Verification items for the finished model (mm, model axes). A direction names the side the tool comes from. Give positions to 0.01 mm unless a question says otherwise; leave off trailing zeros. Order: outer loops, then holes, each group sorted by start corner. A loop starts at its lowest first (then second) coordinate and runs counter-clockwise, first axis right, second up. Notation, with made-up numbers: (63.25, 50.5) -> (109.25, 50.5) arc R22 ccw to (109.25, 82.5) -> close; hole circle Ø7 at (85.5, 61). An arc over 180 degrees is marked (long way). Return JSON: item names as keys, results as strings. Group by question number.
(1) Release check for a two-part mould opening along X. For faces 1 (the face through (104, -14, 0)), 2 (the face through (73, 92.3, 20)) record: pulls with the +X half, pulls with the -X half, needs draft (parallel to the pull), parting line crosses it, or undercut.
(2) Cross-section at B-B on y = -3. Enter the section's corners in (x, z).
(3) Cross-section at A-A on x = 79. Enter the section's corners in (y, z).
(4) Cross-section at C-C on z = 4.5. State how many separate pieces and enclosed holes the cut face has, then the cut area to 3 significant figures.
(5) Tool access check on faces 3 (the face through (118.4, 46, 22)), 4 (the face through (68, 31, 45)). Record the directions out of +Z, -Z, +X, -X, +Y, -Y that give a thin tool (end or side, any length) a straight path to the whole face; none if there is none.
(6) Depth check by flat-ended pin: pin 1 Ø1 at (x, y) = (108.5, 36) entering from +Z. Enter the tip coordinate at first touch or a pass-through.
(7) Thickness scan on line 1 along Y through (x, z) = (73.5, 38); line 2 along X through (y, z) = (68.5, 21.5); line 3 along Z through (x, y) = (43, -6.5). Record the ranges inside material, lowest first.
from build123d import *

# Parameters (mm, degrees)
F1_W     = 152.5
F1_H     = 122.4
F2_DEPTH = 4
F3_DEPTH = 45
F0_W     = 28.1
F0_H     = 28.1
F4_DEPTH = 45.001


with BuildPart() as f2:
    # F1 (on Top) → F2 (new body)
    with BuildSketch(Plane.XY):
        with Locations((74.25, 31.1)):
            Rectangle(F1_W, F1_H)
    extrude(amount=-F2_DEPTH)

    # F1 (on Top) → F3 (join)
    with BuildSketch(Plane.XY):
        with Locations((74.25, 31.1)):
            Rectangle(F1_W, F1_H)
    extrude(amount=F3_DEPTH)

    # F0 (on Top) → F4 (cut, through all)
    with BuildSketch(Plane.XY):
        with Locations((14.05, -14.05)):
            Rectangle(F0_W, F0_H)
        with Locations((14.05, 16.05)):
            Rectangle(F0_W, F0_H)
        with Locations((14.05, 46.15)):
            Rectangle(F0_W, F0_H)
        with Locations((14.05, 76.25)):
            Rectangle(F0_W, F0_H)
        with Locations((44.15, -14.05)):
            Rectangle(F0_W, F0_H)
        with Locations((44.15, 16.05)):
            Rectangle(F0_W, F0_H)
        with Locations((44.15, 46.15)):
            Rectangle(F0_W, F0_H)
        with Locations((44.15, 76.25)):
            Rectangle(F0_W, F0_H)
        with Locations((74.25, -14.05)):
            Rectangle(F0_W, F0_H)
        with Locations((74.25, 16.05)):
            Rectangle(F0_W, F0_H)
        with Locations((74.25, 46.15)):
            Rectangle(F0_W, F0_H)
        with Locations((74.25, 76.25)):
            Rectangle(F0_W, F0_H)
        with Locations((104.35, -14.05)):
            Rectangle(F0_W, F0_H)
        with Locations((104.35, 16.05)):
            Rectangle(F0_W, F0_H)
        with Locations((104.35, 46.15)):
            Rectangle(F0_W, F0_H)
        with Locations((104.35, 76.25)):
            Rectangle(F0_W, F0_H)
        with Locations((134.45, -14.05)):
            Rectangle(F0_W, F0_H)
        with Locations((134.45, 16.05)):
            Rectangle(F0_W, F0_H)
        with Locations((134.45, 46.15)):
            Rectangle(F0_W, F0_H)
        with Locations((134.45, 76.25)):
            Rectangle(F0_W, F0_H)
    extrude(amount=F4_DEPTH, mode=Mode.SUBTRACT)


solid = f2.part
Verdict:
{
 "1": {"face 1": "undercut", "face 2": "needs draft"},
 "2": {"outline": "(-2, -4) -> (150.5, -4) -> (150.5, 45) -> (148.5, 45) -> (148.5, 0) -> (120.4, 0) -> (120.4, 45) -> (118.4, 45) -> (118.4, 0) -> (90.3, 0) -> (90.3, 45) -> (88.3, 45) -> (88.3, 0) -> (60.2, 0) -> (60.2, 45) -> (58.2, 45) -> (58.2, 0) -> (30.1, 0) -> (30.1, 45) -> (28.1, 45) -> (28.1, 0) -> (0, 0) -> (0, 45) -> (-2, 45) -> close"},
 "3": {"outline": "(-30.1, -4) -> (92.3, -4) -> (92.3, 45) -> (90.3, 45) -> (90.3, 0) -> (62.2, 0) -> (62.2, 45) -> (60.2, 45) -> (60.2, 0) -> (32.1, 0) -> (32.1, 45) -> (30.1, 45) -> (30.1, 0) -> (2, 0) -> (2, 45) -> (0, 45) -> (0, 0) -> (-28.1, 0) -> (-28.1, 45) -> (-30.1, 45) -> close"},
 "4": {"separate pieces": "1", "enclosed holes": "20", "area": "2,870 mm²"},
 "5": {"face 3": "+Z", "face 4": "+Z, +X, -X, +Y, -Y"},
 "6": {"pin 1": "z = 0"},
 "7": {"line 1": "-30.1 to -28.1, 0 to 2, 30.1 to 32.1, 60.2 to 62.2, 90.3 to 92.3", "line 2": "-2 to 0, 28.1 to 30.1, 58.2 to 60.2, 88.3 to 90.3, 118.4 to 120.4, 148.5 to 150.5", "line 3": "-4 to 0"}
}
